Input: dimensioned drawing with shaded views. Units: mm. Origin: part minimum x, y, z. Give positions to 0.01 mm unless a question says otherwise; leave off trailing zeros. Write each loop counter-clockwise with the first axis right and the second up, starting at its lowest first coordinate (ties: lowest second). Pieces come first, ordered by that corner, then holes. Notation, with made-up numbers: M -24.5,76 L -10.5,76 A26 cw -10.5,91 Z; hole C -30.75,36.5 d6. An arc over 180 degrees is marked long. Answer as a JSON object with one key per item and string values.
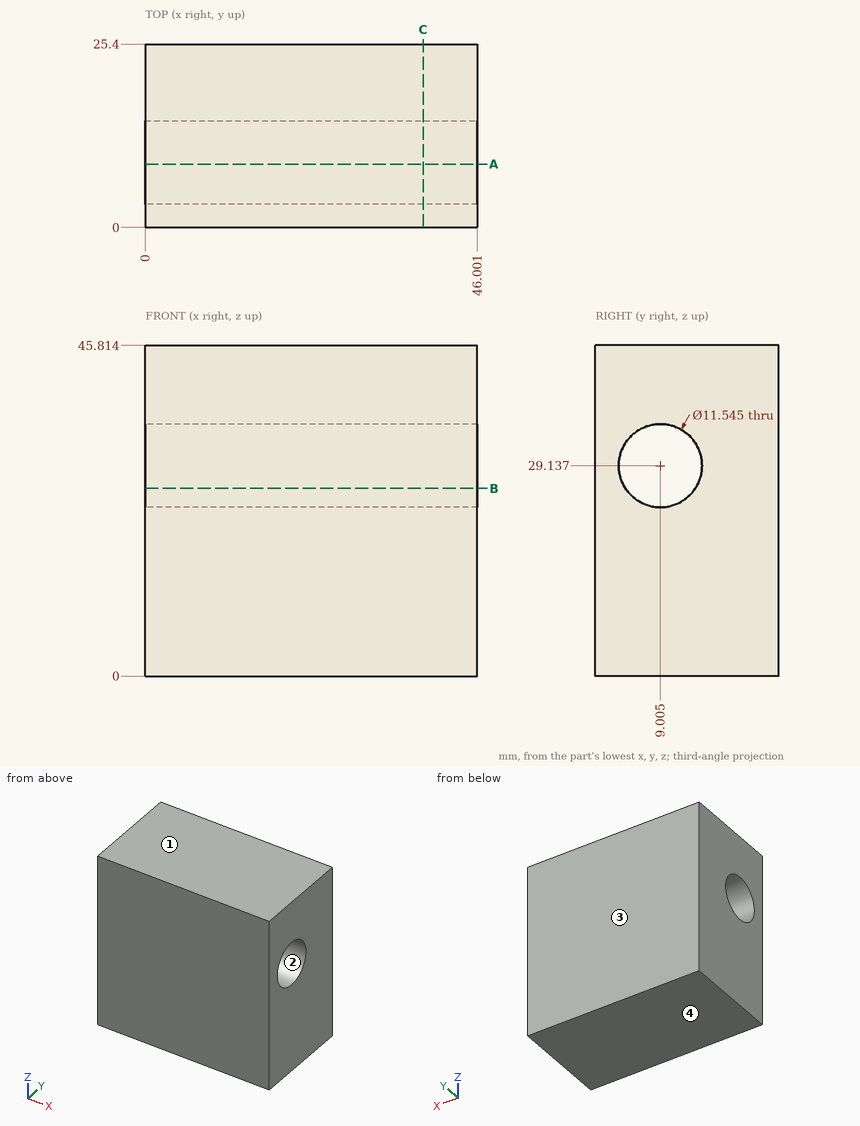
1) Line query: line 1 (Z direction, x = 28, y = 4.75) (1 decimal); line 2 (Y direction, x = 6, z = 31); line 3 (Z direction, x = 42.5, y = 9.5) (1 decimal). Output: solid intervals per line, ascending. Write a range as from..to.
Geometry check:
{"line 1": "z = 0..25.2, 33..45.8", "line 2": "y = 0..3.54, 14.47..25.4", "line 3": "z = 0..23.4, 34.9..45.8"}
2) Cut plane B-B on z = 26. Return loops of the section in (x, y).
Geometry check:
{"outline": "M 0,0 L 46,0 L 46,4.16 L 0,4.16 Z; M 0,13.85 L 46,13.85 L 46,25.4 L 0,25.4 Z"}
3) Pull-direction query (Z, two-part tool) for the marked faces 1, 2, 3 and 4; classes: pulls with the +Z half, pulls with the -Z half, needs draft (parallel to the pull), parting line crosses it, or undercut.
Geometry check:
{"face 1": "pulls with the +Z half", "face 2": "undercut", "face 3": "needs draft", "face 4": "pulls with the -Z half"}
4) Cut plane A-A on y = 8.75. Return loops of the section in (x, z), and give its area (3 significant figures).
Geometry check:
{"outline": "M 0,0 L 46,0 L 46,23.37 L 0,23.37 Z; M 0,34.9 L 46,34.9 L 46,45.81 L 0,45.81 Z", "area": "1,580 mm2"}
5) Cut plane C-C on x = 38.5. Return loops of the section in (y, z) (1 decimal).
Geometry check:
{"outline": "M 0,0 L 25.4,0 L 25.4,45.8 L 0,45.8 Z; hole C 9,29.1 d11.5"}
